Geometry check sheet. Reference: the model listing, model coordinates, mm. Face numbers are marked on the shaded views. Round coordinates to 2 decimals unless told otherwise and drop trailing zeros. Write each loop counter-clockwise with the first axis right and the second up, starting at its lowest first coordinate (ties: lowest second). Pieces come first, ordered by that corner, then holes. Notation, with made-up numbers: (40, -15.75) - (80, -15.75) arc R24 ccw to (80, 20.25) - close; hole circle Ø5 at (27, 58). An arc over 180 degrees is marked (long way). Return JSON: item names as keys, results as strings.
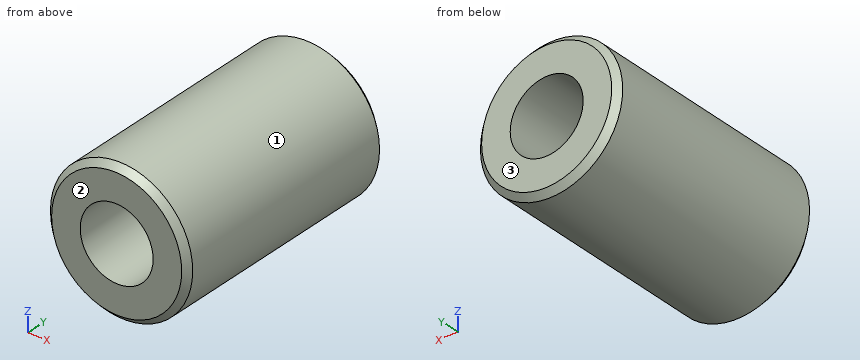
Autodesk Inventor part; units mm, degrees
ref_plane "YZ Plane" through (0, 0, 0) normal (1, 0, 0) x (0, 1, 0)
ref_plane "XZ Plane" through (0, 0, 0) normal (0, 1, 0) x (-1, 0, 0)
ref_plane "XY Plane" through (0, 0, 0) normal (0, 0, 1) x (1, 0, 0)
sketch "Skizze1" plane through (0, 0, 0) normal (0, 1, 0) x (-1, 0, 0)
  circle A0 centre (0, 0) radius 5.85
  dimension "d0" = 11.7
extrude "Extrusion1" add sketch "Skizze1" along normal blind 20
thread "Gewinde1"
sketch "Skizze3" plane through (0, 0, 0) normal (0, -1, 0) x (1, 0, 0)
  circle A0 centre (0, 0) radius 3
  dimension "d5" = 6
extrude "Extrusion2" cut sketch "Skizze3" against normal through all
chamfer "Fase1" distance 0.5 angle 45 2 edges at (5.85, 20, 0) (5.85, 0, 0)
properties part number "Schneckenwelle" material "Messing, weicher Gelbton"
(1) Material ranges on line 1 along Z through (x, y) = (0, 8.25); line 2 along Z through (x, y) = (1, 11); line 3 along Z through (x, y) = (-5, 18), recorded low to high. Write a range as [from, to].
Response values:
{"line 1": "z = [-5.85, -3], [3, 5.85]", "line 2": "z = [-5.76, -2.83], [2.83, 5.76]", "line 3": "z = [-3.04, 3.04]"}
(2) Section check B-B, the plane z = 0. Enter the section's corners in (x, y).
Response values:
{"outline": "(-5.85, 0.5) - (-5.35, 0) - (-3, 0) - (-3, 20) - (-5.35, 20) - (-5.85, 19.5) - close; (3, 0) - (5.35, 0) - (5.85, 0.5) - (5.85, 19.5) - (5.35, 20) - (3, 20) - close"}
(3) Release check for a two-part mould opening along Y. For the marked faces 1, 2 and 3 record: pulls with the +Y half, pulls with the -Y half, needs draft (parallel to the pull), parting line crosses it, or undercut.
Response values:
{"face 1": "needs draft", "face 2": "pulls with the -Y half", "face 3": "pulls with the +Y half"}
(4) Section check A-A, the plane x = 0. Enter the section's corners in (y, z), plus the area to 4 significant figures.
Response values:
{"outline": "(0, -5.35) - (0.5, -5.85) - (19.5, -5.85) - (20, -5.35) - (20, -3) - (0, -3) - close; (0, 3) - (20, 3) - (20, 5.35) - (19.5, 5.85) - (0.5, 5.85) - (0, 5.35) - close", "area": "113.5 mm^2"}
(5) Section check C-C, the plane y = 6.5. Enter the section's corners in (x, z).
Response values:
{"outline": "circle Ø11.7 at (0, 0); hole circle Ø6 at (0, 0)"}
(6) Gauge pin test, flat ends, axial feed: pin 1 (3 mm diameter, centred on x = 4.5, y = 8, fed in from -Z); pin 2 (1.5 mm diameter, centred on y = 8.5, z = 3.5, fed in from +X); pin 3 (6 mm diameter, centred on x = 3.5, y = 13, fed in from +Z); pin 4 (3.5 mm diameter, centred on x = 0, z = 0, fed in from +Y). Record the tip position at first contact, or that the pin passes through.
Response values:
{"pin 1": "stops at z = -5.02", "pin 2": "stops at x = 5.16", "pin 3": "stops at z = 5.83", "pin 4": "passes through"}
